Solid Edge part; units mm, degrees
sketch "Sketch1" plane through (0, 0, 0) normal (0, -1, 0) x (1, 0, 0)
  arc A0 (32.5, 12.5) -> (32.5, -12.5) centre (32.5, 0) cw
  line L0 (-32.5, -12.5) -> (32.5, -12.5)
  arc A1 (-32.5, 12.5) -> (-32.5, -12.5) centre (-32.5, 0) ccw
  line L1 (-32.5, 12.5) -> (32.5, 12.5)
extrude "Protrusion1" add sketch "Sketch1" against normal blind 25.05
hole "Hole_3" at (22.5, 25.05, 0) direction (0, -1, 0) diameter 3.2 depth 3 tip angle 118 start chamfer 0.3 start chamfer angle 45
hole "Hole1" at (-22.5, 25.05, 0) direction (0, -1, 0) diameter 3.2 depth 3 tip angle 118 start chamfer 0.3 start chamfer angle 45
fillet "Round_2" radius 3.5 4 edges at (0, 0, 12.5) (45, 0, 0) (0, 0, -12.5) (-45, 0, 0)
sketch "Sketch2" plane through (0, 0, 0) normal (-1, 0, 0) x (0, -1, 0)
  line L0 (-3.5, 12.5) -> (-25.05, 12.5)
  line L1 (-25.05, 12.5) -> (-25.05, 9)
  line L2 (-25.05, 9) -> (-3.5, 12.5)
  line L3 (-25.05, -9) -> (-3.5, -12.5)
  line L4 (-3.5, -12.5) -> (-25.05, -12.5)
  line L5 (-25.05, -12.5) -> (-25.05, -9)
extrude "ExtrudedCutout_2" cut sketch "Sketch2" along normal mid plane 84
fillet "Round_4" radius 1 4 edges at (0, 25.05, 9) (-45, 25.05, 0) (0, 25.05, -9) (45, 25.05, 0)
sketch "Sketch3" plane through (0, 0, 0) normal (0, -1, 0) x (1, 0, 0)
  circle A0 centre (-32.5, 0) radius 3.5
  circle A1 centre (-11.5, 0) radius 4
  line L0 (-14, -4.5) -> (-9, -4.5)
  arc A2 (-9, -4.5) -> (-4.5, 0) centre (-9, 0) ccw
  arc A3 (-9, 4.5) -> (-4.5, 0) centre (-9, 0) cw
  line L1 (-9, 4.5) -> (-14, 4.5)
  arc A4 (-14, 4.5) -> (-18.5, 0) centre (-14, 0) ccw
  arc A5 (-18.5, 0) -> (-14, -4.5) centre (-14, 0) ccw
  circle A6 centre (17.5, 0) radius 5
  circle A7 centre (32.5, 0) radius 3
extrude "ExtrudedCutout_3" cut sketch "Sketch3" against normal blind 0.1
Here's how the part is built. I have some questions about the finished solid (model axes, mm). A direction names the side the tool comes from. Give positions to 0.01 mm unless a question says otherwise; leave off trailing zeros. Write each loop counter-clockwise with the first axis right and the second up, starting at its lowest first coordinate (ties: lowest second). Pieces come first, ordered by that corner, then holes. Notation, with made-up numbers: (-33, -12) -> (-9, -12) arc R34 ccw to (-9, 20) -> close; hole circle Ø2 at (81.5, -6.75). An arc over 180 degrees is marked (long way). Use one line per item in the form item = value. Start each with the question number.
1. On a 3-axis mill with a long thin cutter (end or side, diameter ignored), from which of +Z, -Z, +X, -X, +Y, -Y can I reach the whole of each face in a straight line? I mean faces 1 (the face through (18, 0.1, 0)), 2 (the face through (-24.086, 23.381, -0.208)), 3 (the face through (0.574, 14, -10.795)). Say none if no direction works.
2. Thinking about a two-plate mould opening in Z: for faces 4 (the face through (20.914, 23.381, -0.208)), 5 (the face through (0.45, 1.05, 11.5)), 6 (the face through (1, 0, 0)), which applies, +Z half, -Z half, draft (parallel to the pull), parting line (faces both ways), or undercut?
3. Will these pins go through, and if not, where does the flat tip stop? pin 1 Ø3 at (x, y) = (32, 14.5) entering from +Z; pin 2 Ø8 at (x, z) = (16.5, 1) entering from -Y; pin 3 Ø4 at (y, z) = (19, 5.5) entering from -X; pin 4 Ø8 at (y, z) = (8.5, -5.5) entering from -X.
4. Imagine slicing it at C-C on y = 16.75. List the corners of the cut face in (x, z) for me.
5. Imagine slicing it at A-A on x = 17.5. List the corners of the cut face in (y, z) for me.
6. If I drill on L1, parallel to X at y = 24.1, z = 0; L2, parallel to Z at x = -22.5, y = 23.7; L3, parallel to X at y = 24.25, z = 2, over which ranges is the centre line in solid material (lowest first)?
7. Imagine slicing it at B-B on y = 8.5. List the corners of the cut face in (x, z) for me.
Entries:
q1.face_1 = -Y
q1.face_2 = +Y
q1.face_3 = -Z, +X, -X, +Y
q2.face_4 = undercut
q2.face_5 = +Z half
q2.face_6 = draft
q3.pin_1 = 10.96
q3.pin_2 = 0
q3.pin_3 = -44.5
q3.pin_4 = -44.91
q4.outline = (-39.51, -10.35) -> (39.51, -10.35) arc R12.5 ccw to (39.51, 10.35) -> (-39.51, 10.35) arc R12.5 ccw to start
q5.outline = (0, -9) arc R3.5 ccw to (3.5, -12.5) -> (24.21, -9.14) arc R1 ccw to (25.05, -8.15) -> (25.05, 8.15) arc R1 ccw to (24.21, 9.14) -> (3.5, 12.5) arc R3.5 ccw to (0, 9) -> (0, 5) -> (0.1, 5) -> (0.1, -5) -> (0, -5) -> close
q6.L1 = -45 to -24.1, -20.9 to 20.9, 24.1 to 45
q6.L2 = -9.22 to -1.6, 1.6 to 9.22
q6.L3 = -44.82 to 44.82
q7.outline = (-36.93, -11.69) -> (36.93, -11.69) arc R12.5 ccw to (36.93, 11.69) -> (-36.93, 11.69) arc R12.5 ccw to start
